Check sheet for the modelled part. Datum: model origin and axes. Units: mm. Round coordinates to 2 decimals unless told otherwise and drop trailing zeros. Loops run counter-clockwise (first coordinate to the right, second up) from the corner with the lowest first, then second, coordinate; pieces in that order, holes last. Notation, with made-up numbers: (76, 39) - (127, 39) arc R21 cw to (127, 43) - close; hole circle Ø4 at (-34, 12). An arc over 180 degrees is marked (long way). Put each result on its own line as item: value.
```python
from build123d import *

# Parameters (mm, degrees)
F1_DEPTH = 152.4
F2_W     = 152.4
F2_H     = 19.05
F3_DEPTH = 19.05


with BuildPart() as f1:
    # F0 (on Front) → F1 (new body, symmetric)
    with BuildSketch(Plane.XZ):
        Polygon((-421.5234547212, 26.9407683632), (-421.5234547212, 0), (189.1339615115, 610.6574162327), (162.1931931483, 610.6574162327), align=None)
    extrude(amount=F1_DEPTH, both=True)

    # F2 (on face) → F3 (cut)
    with BuildSketch(Plane(origin=(-224.2321115422, 0, 224.2321115422), x_dir=(0, -1, 0), z_dir=(-0.7071067812, 0, 0.7071067812))):
        with Locations((-76.2, -199.6370932625)):
            Rectangle(F2_W, F2_H)
        with Locations((-76.2, -91.6870932625)):
            Rectangle(F2_W, F2_H)
        with Locations((-76.2, 16.2629067375)):
            Rectangle(F2_W, F2_H)
        with Locations((-76.2, 124.2129067375)):
            Rectangle(F2_W, F2_H)
        with Locations((-76.2, 232.1629067375)):
            Rectangle(F2_W, F2_H)
        with Locations((-76.2, 340.1129067375)):
            Rectangle(F2_W, F2_H)
        with Locations((-76.2, 448.0629067375)):
            Rectangle(F2_W, F2_H)
    extrude(amount=-F3_DEPTH, mode=Mode.SUBTRACT)


solid = f1.part
```
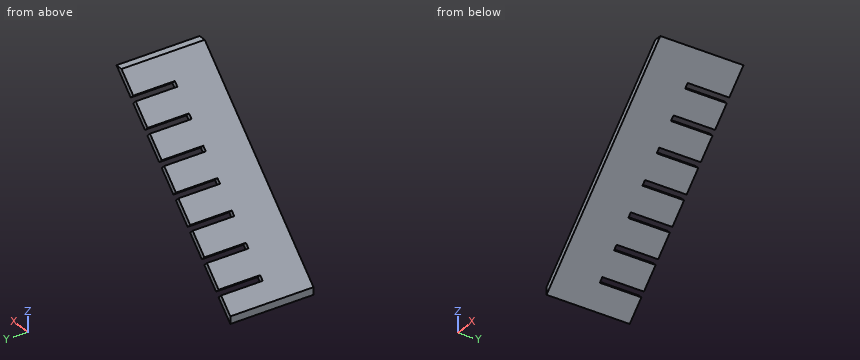
Item 1: Section check B-B on y = -34. Enter the section's corners in (x, z).
Filled sheet:
outline: (-421.52, 0) - (189.13, 610.66) - (162.19, 610.66) - (-421.52, 26.94) - close
Item 2: Section check C-C on x = -82. Enter the section's corners in (y, z), then the cut area to 3 significant figures.
Filled sheet:
outline: (-152.4, 339.52) - (152.4, 339.52) - (152.4, 366.46) - (-152.4, 366.46) - close
area: 8,210 mm²
Item 3: Thickness scan on line 1 (Z direction, x = -327.5, y = -99); line 2 (X direction, y = -39, z = 565.5); line 3 (X direction, y = 72, z = 369). Record the ranges inside material, lowest first. Write a range as from..to.
Filled sheet:
line 1: 94.02..120.96
line 2: 117.04..143.98
line 3: -79.46..-54.14
Item 4: Go/stop test with flat-tipped pins: pin 1 (8 mm diameter, centred on x = 122.5, y = 16.5, fed in from -Z); pin 2 (1 mm diameter, centred on y = -11, z = 296.5, fed in from -X); pin 3 (8 mm diameter, centred on x = -276, z = 149.5, fed in from +Y). Record where each tip stops, or that it passes through.
Filled sheet:
pin 1: z = 540.02
pin 2: x = -152.46
pin 3: y = 0
Item 5: Section check A-A on y = 42. Count the separate pieces of the cut face and the enclosed holes in it, then the cut area to 3 significant figures.
Filled sheet:
separate pieces: 8
enclosed holes: 0
area: 13,500 mm²
